```python
from build123d import *

# Parameters (mm, degrees)
SKETCH1_W           = 75
SKETCH1_H           = 12
SKETCH1_R           = 11
SKETCH1_R_2         = 2.5
BOSS_EXTRUDE1_DEPTH = 10
FILLET1_R           = 4
FILLET2_R           = 12
FILLET3_R           = 10


with BuildPart() as part:
    # Sketch1 → Boss-Extrude1 (new body)
    with BuildSketch(Plane(origin=(0, 0, 0), x_dir=(1, 0, 0), z_dir=(0, 1, 0))):
        with BuildLine():
            ThreePointArc((12.737739203, 12), (-17.5, 0), (12.737739203, -12))
            Line((12.737739203, -12), (207.262260797, -12))
            ThreePointArc((207.262260797, -12), (233.974449241, -10.533981603), (228.029081208, 15.549400469))
            Line((228.029081208, 15.549400469), (233.534736894, 26.211846505))
            Line((233.534736894, 26.211846505), (249.534736894, 35.402238979))
            Line((249.534736894, 35.402238979), (256.413650124, 48.724183776))
            ThreePointArc((256.413650124, 48.724183776), (256.734536929, 52.537540906), (254.264987478, 55.460892826))
            Line((254.264987478, 55.460892826), (245.379615782, 60.048939231))
            ThreePointArc((245.379615782, 60.048939231), (241.566258652, 60.369826035), (238.642906731, 57.900276585))
            Line((238.642906731, 57.900276585), (233.596055686, 48.126367719))
            ThreePointArc((233.596055686, 48.126367719), (226.580011076, 42.199449038), (217.427953964, 42.969577368))
            Line((217.427953964, 42.969577368), (215.650879625, 43.887186649))
            ThreePointArc((215.650879625, 43.887186649), (209.549508217, 44.400605536), (204.872145144, 40.449326415))
            Line((204.872145144, 40.449326415), (197.072466256, 25.344194531))
            Line((197.072466256, 25.344194531), (197.072466256, 12))
            Line((197.072466256, 12), (12.737739203, 12))
        make_face()
        with Locations((65, 0)):
            Rectangle(SKETCH1_W, SKETCH1_H, mode=Mode.SUBTRACT)
        with Locations((155, 0)):
            Rectangle(SKETCH1_W, SKETCH1_H, mode=Mode.SUBTRACT)
        Circle(SKETCH1_R, mode=Mode.SUBTRACT)
        with Locations((244.775450585, 47.981007162)):
            Circle(SKETCH1_R_2, mode=Mode.SUBTRACT)
        Polygon((207.392396097, 27.893517595), (211.980442501, 36.778889292), (219.088739859, 33.108452168), (214.500693454, 24.223080471), align=None, mode=Mode.SUBTRACT)
        with Locations((220, 0)):
            Circle(SKETCH1_R, mode=Mode.SUBTRACT)
    extrude(amount=BOSS_EXTRUDE1_DEPTH)

    # Fillet1
    fillet1_edges = [part.edges().sort_by_distance(p)[0] for p in [
        (27.5, 5, -6),
        (27.5, 5, 6),
        (102.5, 5, 6),
        (102.5, 5, -6),
        (117.5, 5, -6),
        (117.5, 5, 6),
        (192.5, 5, 6),
        (192.5, 5, -6),
    ]]
    fillet(fillet1_edges, radius=FILLET1_R)

    # Fillet2
    fillet2_edges = [part.edges().sort_by_distance(p)[0] for p in [
        (12.737739203, 5, 12),
        (12.737739203, 5, -12),
        (207.262260797, 5, 12),
    ]]
    fillet(fillet2_edges, radius=FILLET2_R)

    # Fillet3
    fillet3_edges = [part.edges().sort_by_distance(p)[0] for p in [
        (197.072466256, 5, -12),
        (197.072466256, 5, -25.344194531),
        (249.534736894, 5, -35.402238979),
        (233.534736894, 5, -26.211846505),
        (228.029081208, 5, -15.549400469),
    ]]
    fillet(fillet3_edges, radius=FILLET3_R)


solid = part.part
```
Input: part model. Units: mm. Frame: model coordinates. A direction names the side the tool comes from. Round coordinates to 2 decimals unless told otherwise and drop trailing zeros. Loops run counter-clockwise (first coordinate to the right, second up) from the corner with the lowest first, then second, coordinate; pieces in that order, holes last. Notation, with made-up numbers: (73.25, 21) -> (132.25, 21) arc R17 cw to (132.25, 36) -> close; hole circle Ø6 at (41, -28.75). An arc over 180 degrees is marked (long way). Use one line per item in the form item = value. Start each with the question number.
Item 1: Section query A-A on x = 46. Return the cut outline in (y, z), then the cut area to 3 significant figures.
Item 2: Set-up query: faces 1 (the face through (211, 4.93, -26.03)), 2 (the face through (194.065, 5.07, -14.852)), 3 (the face through (201.58, 4.93, -34.07)). Return all of +Z, -Z, +X, -X, +Y, -Y with unobstructed straight access to the full face (end or side cutting, diameter ignored); none if empty.
Item 3: Contact query for flat-ended pins moving along their axis: pin 1 Ø1 at (y, z) = (7, -20.5) entering from +X; pin 2 Ø2 at (y, z) = (6.5, 0) entering from +X; pin 3 Ø5 at (y, z) = (7.5, -44) entering from -X. Output: stop coordinate, or through.
Item 4: Mould query, pull axis Z, two halves, no side actions, for faces 4 (the face through (139, 0, -7)), 5 (the face through (65, 5, -6)), 6 (the face through (13.44, 5.07, -12.59)). Classes: pulls with the +Z half, pulls with the -Z half, needs draft (parallel to the pull), parting line crosses it, or undercut.
Item 5: Section query C-C on y = 4.75. Count the separate pieces of the cut face and the enclosed holes in it, then the cut area to 3 significant figures.
Item 6: Material intervals for L1, parallel to X at y = 7, z = 0; L2, parallel to Z at x = 45, y = 8.25; L3, parallel to Z at x = 0, y = 5.5, sorted ascending. Write a range as from..to.
Item 7: Section query B-B on x = 0. Return the cut outline in (y, z), then the cut area to 3 significant figures.
Item 8: Section query D-D on x = 106. Return the cut outline in (y, z), then the cut area to 3 significant figures.
Ans:
q1.outline = (0, -12) -> (10, -12) -> (10, -6) -> (0, -6) -> close; (0, 6) -> (10, 6) -> (10, 12) -> (0, 12) -> close
q1.area = 120 mm^2
q2.face_1 = +Y, -Y
q2.face_2 = -Z, +Y, -Y
q2.face_3 = -Z, -X, +Y, -Y
q3.pin_1 = 231.05
q3.pin_2 = 237.5
q3.pin_3 = 205.52
q4.face_4 = needs draft
q4.face_5 = undercut
q4.face_6 = pulls with the -Z half
q5.separate_pieces = 1
q5.enclosed_holes = 6
q5.area = 5,290 mm^2
q6.L1 = -17.5..-11, 11..27.5, 102.5..117.5, 192.5..209, 231..237.5
q6.L2 = -12..-6, 6..12
q6.L3 = -17.5..-11, 11..17.5
q7.outline = (0, -17.5) -> (10, -17.5) -> (10, -11) -> (0, -11) -> close; (0, 11) -> (10, 11) -> (10, 17.5) -> (0, 17.5) -> close
q7.area = 130 mm^2
q8.outline = (0, -12) -> (10, -12) -> (10, 12) -> (0, 12) -> close
q8.area = 240 mm^2
